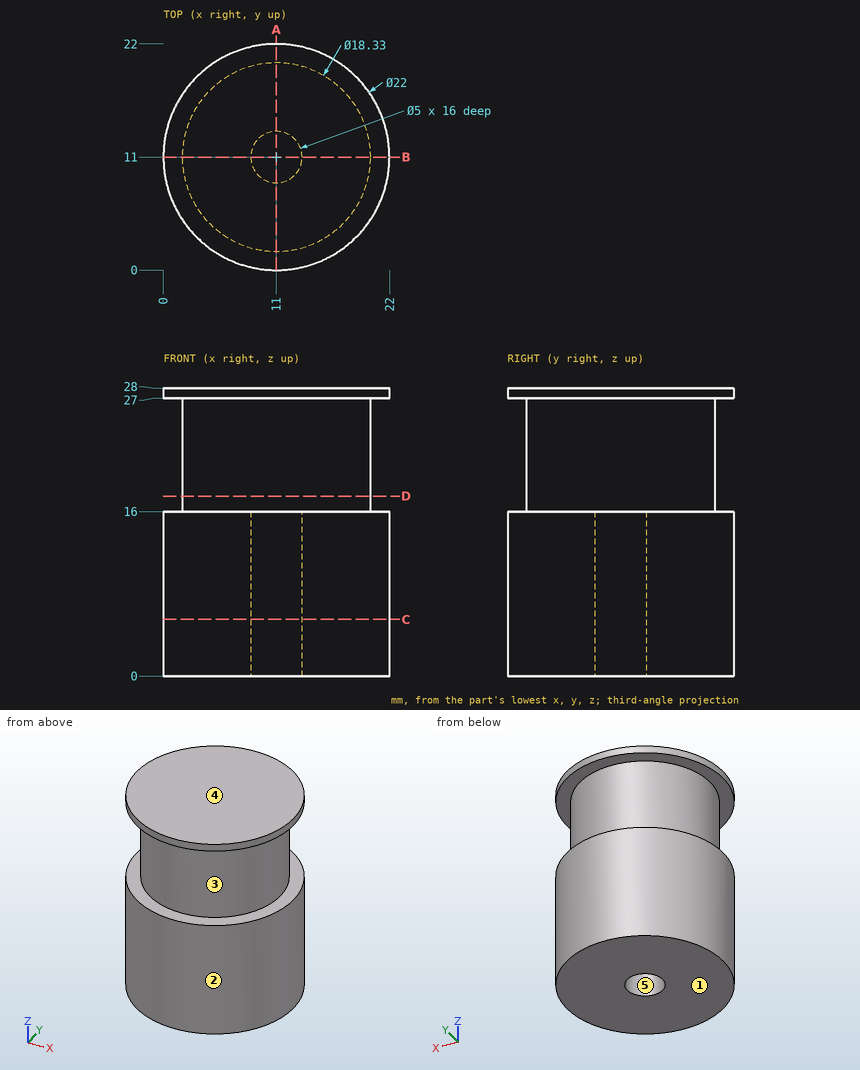
Verification items for this drawing (mm, ordinates from the low corner). A direction names the side the tool comes from. Give positions to 0.01 mm unless a question says otherwise; leave off trailing zeros. Write each loop counter-clockwise with the first axis right and the second up, starting at its lowest first coordinate (ties: lowest second). Pieces come first, ordered by that corner, then holes.
1) Set-up check for the marked faces 4 and 5: record each of +Z, -Z, +X, -X, +Y, -Y from which the full face is reachable in a straight line by a thin tool's end or side.
Values follow:
face 4: +Z, +X, -X, +Y, -Y
face 5: -Z
2) Cross-section at C-C (z = 5.5). Record the boundary of the cut face in (x, y), plus the area to 3 significant figures.
Values follow:
outline: circle Ø22 at (11, 11); hole circle Ø5 at (11, 11)
area: 360 mm2
3) Release check for a two-part mould opening along Z. For the marked faces 1, 2 and 3 record: released by +Z, released by -Z, zero draft, split by the parting line, or undercut.
Values follow:
face 1: released by -Z
face 2: zero draft
face 3: undercut
4) Go/stop test with flat-tipped pins: pin 1 Ø4 at (x, z) = (5.5, 22.5) entering from -Y; pin 2 Ø6 at (x, z) = (5, 14) entering from +Y; pin 3 Ø1.5 at (x, y) = (9, 11) entering from -Z; pin 4 Ø3 at (x, z) = (16, 4.5) entering from +Y. Record where each tip stops, or that it passes through.
Values follow:
pin 1: stops at y = 2.53
pin 2: stops at y = 21.58
pin 3: stops at z = 0
pin 4: stops at y = 21.43
5) Cross-section at A-A (x = 11). Record the boundary of the cut face in (y, z) (3 decimals), plus the area to 3 significant figures.
Values follow:
outline: (0, 0) - (8.5, 0) - (8.5, 16) - (13.5, 16) - (13.5, 0) - (22, 0) - (22, 16) - (20.165, 16) - (20.165, 27) - (22, 27) - (22, 28) - (0, 28) - (0, 27) - (1.835, 27) - (1.835, 16) - (0, 16) - close
area: 496 mm2
6) Thickness scan on line 1 (Y direction, x = 11, z = 4.75); line 2 (Z direction, x = 2, y = 6.75); line 3 (X direction, y = 9.5, z = 1.75). Record the ranges inside material, lowest first.
Values follow:
line 1: y = 0 to 8.5, 13.5 to 22
line 2: z = 0 to 16, 27 to 28
line 3: x = 0.1 to 9, 13 to 21.9
7) Cross-section at D-D (z = 17.5). Record the boundary of the cut face in (x, y) (3 decimals), plus the area to 3 significant figures.
Values follow:
outline: circle Ø18.33 at (11, 11)
area: 264 mm2
